```python
from build123d import *

# Parameters (mm, degrees)
CROQUIS2_W              = 60
CROQUIS2_H              = 60
CROQUIS2_W_2            = 50
CROQUIS2_H_2            = 50
SALIENTE_EXTRUIR1_DEPTH = 10
CROQUIS3_W              = 60
CROQUIS3_H              = 5
SALIENTE_EXTRUIR2_DEPTH = 170
CROQUIS5_W              = 10
CROQUIS5_H              = 60
SALIENTE_EXTRUIR3_DEPTH = 55
CROQUIS7_W              = 50
CROQUIS7_H              = 50.027491106
CORTAR_EXTRUIR1_DEPTH   = 10
CROQUIS8_W              = 160
CROQUIS8_H              = 5
CORTAR_EXTRUIR2_DEPTH   = 10


with BuildPart() as part:
    # Croquis2 → Saliente-Extruir1 (new body)
    with BuildSketch(Plane(origin=(0, 0, 0), x_dir=(0, 0, -1), z_dir=(1, 0, 0))):
        with Locations((0, 0.130518683)):
            Rectangle(CROQUIS2_W, CROQUIS2_H)
        with Locations((0, 0.130518683)):
            Rectangle(CROQUIS2_W_2, CROQUIS2_H_2, mode=Mode.SUBTRACT)
    extrude(amount=SALIENTE_EXTRUIR1_DEPTH)

    # Croquis3 → Saliente-Extruir2 (add)
    with BuildSketch(Plane(origin=(10, 0, 0), x_dir=(0, 0, -1), z_dir=(1, 0, 0))):
        with Locations((0, 27.630518683)):
            Rectangle(CROQUIS3_W, CROQUIS3_H)
    extrude(amount=SALIENTE_EXTRUIR2_DEPTH)

    # Croquis5 → Saliente-Extruir3 (add)
    with BuildSketch(Plane.XZ.offset(-25.130518683)):
        with Locations((175, 0)):
            Rectangle(CROQUIS5_W, CROQUIS5_H)
    extrude(amount=SALIENTE_EXTRUIR3_DEPTH)

    # Croquis7 → Cortar-Extruir1 (cut)
    with BuildSketch(Plane(origin=(180, 0, 0), x_dir=(0, 0, -1), z_dir=(1, 0, 0))):
        with Locations((0, 0.144264236)):
            Rectangle(CROQUIS7_W, CROQUIS7_H)
    extrude(amount=-CORTAR_EXTRUIR1_DEPTH, mode=Mode.SUBTRACT)

    # Croquis8 → Cortar-Extruir2 (cut)
    with BuildSketch(Plane(origin=(0, 30.130518683, 0), x_dir=(1, 0, 0), z_dir=(0, 1, 0))):
        with Locations((90, 12.5)):
            Rectangle(CROQUIS8_W, CROQUIS8_H)
        with Locations((90, -12.5)):
            Rectangle(CROQUIS8_W, CROQUIS8_H)
    extrude(amount=-CORTAR_EXTRUIR2_DEPTH, mode=Mode.SUBTRACT)


solid = part.part
```
Verification items for the finished model (mm, model axes). A direction names the side the tool comes from. Coordinates: 2 decimals unless noted, no trailing zeros. Loops run counter-clockwise (first coordinate to the right, second up) from the corner with the lowest first, then second, coordinate; pieces in that order, holes last. Notation, with made-up numbers: (-20.75, 42) -> (31.25, 42) arc R21 ccw to (31.25, 70) -> close; hole circle Ø4 at (-26, -8). An arc over 180 degrees is marked (long way). Answer in a Markdown table with one row per item.
1) Section check D-D (y = -9). Record the cut outline in (x, z), and give its area (3 significant figures).
The answers:
| item | result |
|---|---|
| outline | (0, -30) -> (10, -30) -> (10, -25) -> (0, -25) -> close; (0, 25) -> (10, 25) -> (10, 30) -> (0, 30) -> close; (170, -30) -> (180, -30) -> (180, -25) -> (170, -25) -> close; (170, 25) -> (180, 25) -> (180, 30) -> (170, 30) -> close |
| area | 200 mm2 |
2) Section check B-B (z = -12.5). Record the cut outline in (x, y).
The answers:
| item | result |
|---|---|
| outline | (0, -29.87) -> (10, -29.87) -> (10, -24.87) -> (0, -24.87) -> close; (0, 25.13) -> (10, 25.13) -> (10, 30.13) -> (0, 30.13) -> close; (170, -29.87) -> (180, -29.87) -> (180, -24.87) -> (170, -24.87) -> close; (170, 25.16) -> (180, 25.16) -> (180, 30.13) -> (170, 30.13) -> close |
3) Depth check by flat-ended pin: P1, Ø4, axis at x = 21, z = 2.5, coming from the -Y side. Enter the tip coordinate at first touch or a pass-through.
The answers:
| item | result |
|---|---|
| P1 | stops at y = 25.13 |
4) Scan lines: line 1 along X through (y, z) = (-23.5, 25.5); line 2 along Y through (x, z) = (103, -23). Record each from-to range of solid material in increasing order. Write a range as from..to.
The answers:
| item | result |
|---|---|
| line 1 | x = 0..10, 170..180 |
| line 2 | y = 25.13..30.13 |
5) Section check A-A (x = 101.5). Record the cut outline in (y, z), and give its area (3 significant figures).
The answers:
| item | result |
|---|---|
| outline | (25.13, -30) -> (30.13, -30) -> (30.13, -15) -> (25.13, -15) -> close; (25.13, -10) -> (30.13, -10) -> (30.13, 10) -> (25.13, 10) -> close; (25.13, 15) -> (30.13, 15) -> (30.13, 30) -> (25.13, 30) -> close |
| area | 250 mm2 |
6) Draft check along X on faces 1 (the face through (89, 28, -10)), 2 (the face through (5, -29.869, 0)), 3 (the face through (0, 1, 27)). Enter one of: released by +X, released by -X, zero draft, split by the parting line, or undercut.
The answers:
| item | result |
|---|---|
| face 1 | undercut |
| face 2 | zero draft |
| face 3 | released by -X |
7) Section check C-C (z = 1.5). Give the number of separate pieces and of enclosed holes in the cut face, and give its area (4 significant figures).
The answers:
| item | result |
|---|---|
| separate pieces | 3 |
| enclosed holes | 0 |
| area | 1,000 mm2 |
8) Access from +Z, -Z, +X, -X, +Y, -Y to the whole of each face (thin tool, end or side, straight path). Record for faces 4 (the face through (170, -27, 0)), 5 (the face through (5, 0, -25)), 6 (the face through (89, 30.131, 0)), 7 (the face through (70, 27, -30)), 8 (the face through (10, 28, -12)).
The answers:
| item | result |
|---|---|
| face 4 | +Z, -Z, -Y |
| face 5 | +X, -X |
| face 6 | +Z, -Z, +X, -X, +Y |
| face 7 | -Z, +X, -X, +Y, -Y |
| face 8 | +Y, -Y |
